from build123d import *

# Parameters (mm, degrees)
SKETCH_1_W          = 20
SKETCH_1_H          = 20
SKETCH_1_W_2        = 18
SKETCH_1_H_2        = 18
EXTRUDE_1_DEPTH     = 171.98
SKETCH_2_R          = 1.5
CUT_EXTRUDE_1_DEPTH = 50
SKETCH_4_W          = 20
SKETCH_4_H          = 8.4
CUT_EXTRUDE_2_DEPTH = 21
SKETCH_5_R          = 2.5
CUT_EXTRUDE_3_DEPTH = 36
SKETCH_6_W          = 20
SKETCH_6_H          = 3
CUT_EXTRUDE_4_DEPTH = 33


with BuildPart() as part:
    # 草图1 → 凸台-拉伸1 (new body)
    with BuildSketch(Plane.XY):
        Rectangle(SKETCH_1_W, SKETCH_1_H)
        Rectangle(SKETCH_1_W_2, SKETCH_1_H_2, mode=Mode.SUBTRACT)
    extrude(amount=EXTRUDE_1_DEPTH)

    # 草图2 → 切除-拉伸1 (cut)
    with BuildSketch(Plane(origin=(0, 10, 0), x_dir=(1, 0, 0), z_dir=(0, 1, 0))):
        with Locations((-5, -5)):
            Circle(SKETCH_2_R)
        with Locations((5, -5)):
            Circle(SKETCH_2_R)
        with Locations((-5, -15)):
            Circle(SKETCH_2_R)
        with Locations((5, -15)):
            Circle(SKETCH_2_R)
        with Locations((-5, -235)):
            Circle(SKETCH_2_R)
        with Locations((5, -245)):
            Circle(SKETCH_2_R)
        with Locations((5, -235)):
            Circle(SKETCH_2_R)
        with Locations((-5, -245)):
            Circle(SKETCH_2_R)
    extrude(amount=-CUT_EXTRUDE_1_DEPTH, mode=Mode.SUBTRACT)

    # 草图4 → 切除-拉伸2 (cut, through all)
    with BuildSketch(Plane.XZ.offset(10)):
        with Locations((0, 167.78)):
            Rectangle(SKETCH_4_W, SKETCH_4_H)
    extrude(amount=-CUT_EXTRUDE_2_DEPTH, mode=Mode.SUBTRACT)

    # 草图5 → 切除-拉伸3 (cut)
    with BuildSketch(Plane(origin=(0, 10, 0), x_dir=(1, 0, 0), z_dir=(0, 1, 0))):
        with Locations((0, -153.58)):
            Circle(SKETCH_5_R)
        with Locations((0, -133.26)):
            Circle(SKETCH_5_R)
    extrude(amount=-CUT_EXTRUDE_3_DEPTH, mode=Mode.SUBTRACT)

    # 草图6 → 切除-拉伸4 (cut)
    with BuildSketch(Plane(origin=(0, 10, 0), x_dir=(1, 0, 0), z_dir=(0, 1, 0))):
        with Locations((0, -162.08)):
            Rectangle(SKETCH_6_W, SKETCH_6_H)
    extrude(amount=-CUT_EXTRUDE_4_DEPTH, mode=Mode.SUBTRACT)


solid = part.part
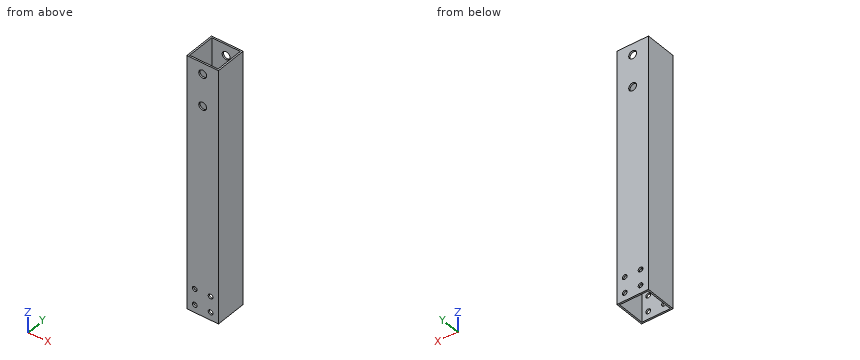
Model file for the job. Use its own axes, mm. Give positions to 0.01 mm unless a question says otherwise; leave off trailing zeros. Loops run counter-clockwise (first coordinate to the right, second up) from the corner with the lowest first, then second, coordinate; pieces in that order, holes last.
Item 1: Drill centre lines: line 1 along X through (y, z) = (9.6, 15); line 2 along X through (y, z) = (4.75, 108.5); line 3 along Z through (x, y) = (0, -9.6). Where is each one in solid material? Low to high.
Check values:
line 1: x = -10 to -6.5, -3.5 to 3.5, 6.5 to 10
line 2: x = -10 to -9, 9 to 10
line 3: z = 0 to 130.76, 135.76 to 151.08, 156.08 to 160.58
Item 2: Slice it at B-B (z = 153.58). Write the cut outline in (x, y).
Check values:
outline: (-10, -10) - (-2.5, -10) - (-2.5, -9) - (-9, -9) - (-9, 9) - (-2.5, 9) - (-2.5, 10) - (-10, 10) - close; (2.5, -10) - (10, -10) - (10, 10) - (2.5, 10) - (2.5, 9) - (9, 9) - (9, -9) - (2.5, -9) - close
Item 3: Slice it at C-C (y = 4.25). Write the cut outline in (x, z).
Check values:
outline: (-10, 0) - (-9, 0) - (-9, 160.58) - (-10, 160.58) - close; (9, 0) - (10, 0) - (10, 160.58) - (9, 160.58) - close
Item 4: Slice it at A-A (x = -5). Write the cut outline in (y, z).
Check values:
outline: (-10, 0) - (-9, 0) - (-9, 3.5) - (-10, 3.5) - close; (-10, 6.5) - (-9, 6.5) - (-9, 13.5) - (-10, 13.5) - close; (-10, 16.5) - (-9, 16.5) - (-9, 160.58) - (-10, 160.58) - close; (9, 0) - (10, 0) - (10, 3.5) - (9, 3.5) - close; (9, 6.5) - (10, 6.5) - (10, 13.5) - (9, 13.5) - close; (9, 16.5) - (10, 16.5) - (10, 160.58) - (9, 160.58) - close
Item 5: Slice it at D-D (z = 50). Write the cut outline in (x, y).
Check values:
outline: (-10, -10) - (10, -10) - (10, 10) - (-10, 10) - close; hole (-9, -9) - (9, -9) - (9, 9) - (-9, 9) - close
